The model under review builds one solid part; all positions refer to its coordinate system, in mm. Round coordinates to 2 decimals unless told otherwise and drop trailing zeros. Loops run counter-clockwise (first coordinate to the right, second up) from the corner with the lowest first, then second, coordinate; pieces in that order, holes last. Notation, with made-up numbers: (65.25, 47) -> (95.25, 47) arc R20 cw to (95.25, 51) -> close; hole circle Ø11 at (17.5, -1). An arc over 180 degrees is marked (long way). Write each question's results on one line, items separated by ' | '. Start each with the question number.
Item 1: Clearance check with flat-ended pins moving along their axes: pin 1 Ø0.5 at (x, z) = (0.5, 0.5) entering from +Y; pin 2 Ø0.9 at (x, z) = (15, 2) entering from -Y; pin 3 Ø0.9 at (x, z) = (-1, 2) entering from +Y. State where each tip first meets the part, or that it passes through.
Item 2: We need section D-D (y = -3.25). Give the boundary of the cut face in (x, z), and give its area (3 significant figures).
Item 3: We need section C-C (x = 11). Give the boundary of the cut face in (y, z).
Item 4: We need section A-A (y = 1). Give the boundary of the cut face in (x, z).
Item 5: For L1, parallel to Z at x = 20, y = 2; L2, parallel to X at y = 0.75, z = 1.15; L3, parallel to X at y = -0.25, z = 1.3, list the stretches that pass through material, from the lowest coordinate up. Write a range as from..to.
Item 6: We need section B-B (x = 15.25). Give the boundary of the cut face in (y, z).
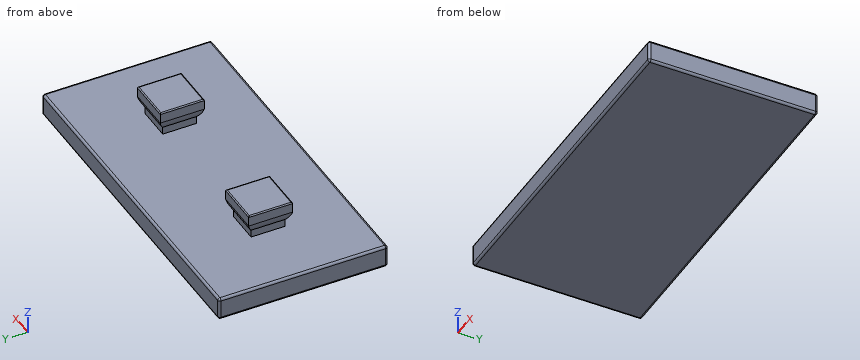
from build123d import *

# Parameters (mm, degrees)
SKETCH_1_W                      = 30
SKETCH_1_H                      = 15
EXTRUDE_1_DEPTH                 = 2
SKETCH_2_W                      = 3
SKETCH_2_H                      = 3
EXTRUDE_2_DEPTH                 = 1
EXTRUDE_3_DEPTH                 = 2
CUT_EXTRUDE_1_REACH             = 25.848
CUT_EXTRUDE_1_DIRECTION_2_REACH = 25.848
FILLET_1_R                      = 0.1
FILLET_1_OF_MIRROR_1_R          = 0.1
FILLET_3_R                      = 0.2


with BuildPart() as part:
    # Sketch 1 → Extrude 1 (new body)
    with BuildSketch(Plane.XY):
        with Locations((7.5, 0)):
            Rectangle(SKETCH_1_W, SKETCH_1_H)
    extrude(amount=-EXTRUDE_1_DEPTH)

    # Sketch 2 → Extrude 2 (add)
    with BuildSketch(Plane.XY):
        Rectangle(SKETCH_2_W, SKETCH_2_H)
    extrude_2 = extrude(amount=EXTRUDE_2_DEPTH)

    # Sketch 3 → Extrude 3 (add, symmetric)
    with BuildSketch(Plane(origin=(0, 0, 0), x_dir=(1, 0, 0), z_dir=(0, 1, 0))):
        with BuildLine():
            Line((-1.95, -2.5), (1.95, -2.5))
            Line((1.95, -2.5), (1.95, -1.555590279))
            ThreePointArc((1.95, -1.555590279), (1.780042303, -1.088161527), (1.5, -0.677124344))
            Line((1.5, -0.677124344), (-1.5, -0.677124344))
            ThreePointArc((-1.5, -0.677124344), (-1.780042303, -1.088161527), (-1.95, -1.555590279))
            Line((-1.95, -1.555590279), (-1.95, -2.5))
        make_face()
    extrude_3 = extrude(amount=EXTRUDE_3_DEPTH, both=True)

    # Sketch 4 → Cut-Extrude 1 (cut, up to next)
    with BuildSketch(Plane(origin=(0, 0, 0), x_dir=(0, 0, -1), z_dir=(1, 0, 0)), mode=Mode.PRIVATE) as cut_extrude_1_sk1:
        with BuildLine():
            Line((-2.5, 1.95), (-1.555590279, 1.95))
            ThreePointArc((-1.555590279, 1.95), (-1.088161527, 1.780042303), (-0.677124344, 1.5))
            Line((-0.677124344, 1.5), (-0.677124344, 2))
            Line((-0.677124344, 2), (-2.5, 2))
            Line((-2.5, 2), (-2.5, 1.95))
        make_face()
    cut_extrude_1_tool1 = extrude(cut_extrude_1_sk1.sketch, amount=-CUT_EXTRUDE_1_REACH, mode=Mode.PRIVATE) & part.part
    # Sketch 4 → Cut-Extrude 1 (cut, up to next)
    with BuildSketch(Plane(origin=(0, 0, 0), x_dir=(0, 0, -1), z_dir=(1, 0, 0)), mode=Mode.PRIVATE) as cut_extrude_1_sk2:
        with BuildLine():
            Line((-2.5, -2), (-0.677124344, -2))
            Line((-0.677124344, -2), (-0.677124344, -1.5))
            ThreePointArc((-0.677124344, -1.5), (-1.088161527, -1.780042303), (-1.555590279, -1.95))
            Line((-1.555590279, -1.95), (-2.5, -1.95))
            Line((-2.5, -1.95), (-2.5, -2))
        make_face()
    cut_extrude_1_tool2 = extrude(cut_extrude_1_sk2.sketch, amount=-CUT_EXTRUDE_1_REACH, mode=Mode.PRIVATE) & part.part
    cut_extrude_1_1 = cut_extrude_1_tool1.solids().sort_by_distance((0, 1.873038, 1.175075))[0]
    add(cut_extrude_1_1, mode=Mode.SUBTRACT)
    cut_extrude_1_2 = cut_extrude_1_tool2.solids().sort_by_distance((0, -1.873038, 1.175075))[0]
    add(cut_extrude_1_2, mode=Mode.SUBTRACT)
    cut_extrude_1 = cut_extrude_1_1 + cut_extrude_1_2  # Cut-Extrude 1 as one shape, for the pattern or mirror that repeats it

    # Sketch 4 → Cut-Extrude 1 direction 2 (cut, up to next)
    with BuildSketch(Plane(origin=(0, 0, 0), x_dir=(0, 0, -1), z_dir=(1, 0, 0)), mode=Mode.PRIVATE) as cut_extrude_1_direction_2_sk1:
        with BuildLine():
            Line((-2.5, 1.95), (-1.555590279, 1.95))
            ThreePointArc((-1.555590279, 1.95), (-1.088161527, 1.780042303), (-0.677124344, 1.5))
            Line((-0.677124344, 1.5), (-0.677124344, 2))
            Line((-0.677124344, 2), (-2.5, 2))
            Line((-2.5, 2), (-2.5, 1.95))
        make_face()
    cut_extrude_1_direction_2_tool1 = extrude(cut_extrude_1_direction_2_sk1.sketch, amount=CUT_EXTRUDE_1_DIRECTION_2_REACH, mode=Mode.PRIVATE) & part.part
    # Sketch 4 → Cut-Extrude 1 direction 2 (cut, up to next)
    with BuildSketch(Plane(origin=(0, 0, 0), x_dir=(0, 0, -1), z_dir=(1, 0, 0)), mode=Mode.PRIVATE) as cut_extrude_1_direction_2_sk2:
        with BuildLine():
            Line((-2.5, -2), (-0.677124344, -2))
            Line((-0.677124344, -2), (-0.677124344, -1.5))
            ThreePointArc((-0.677124344, -1.5), (-1.088161527, -1.780042303), (-1.555590279, -1.95))
            Line((-1.555590279, -1.95), (-2.5, -1.95))
            Line((-2.5, -1.95), (-2.5, -2))
        make_face()
    cut_extrude_1_direction_2_tool2 = extrude(cut_extrude_1_direction_2_sk2.sketch, amount=CUT_EXTRUDE_1_DIRECTION_2_REACH, mode=Mode.PRIVATE) & part.part
    cut_extrude_1_direction_2_1 = cut_extrude_1_direction_2_tool1.solids().sort_by_distance((0, 1.873038, 1.175075))[0]
    add(cut_extrude_1_direction_2_1, mode=Mode.SUBTRACT)
    cut_extrude_1_direction_2_2 = cut_extrude_1_direction_2_tool2.solids().sort_by_distance((0, -1.873038, 1.175075))[0]
    add(cut_extrude_1_direction_2_2, mode=Mode.SUBTRACT)
    cut_extrude_1_direction_2 = cut_extrude_1_direction_2_1 + cut_extrude_1_direction_2_2  # Cut-Extrude 1 direction 2 as one shape, for the pattern or mirror that repeats it

    # Fillet 1
    fillet_1_edges = [part.edges().sort_by_distance(p)[0] for p in [
        (-1.95, 0, 2.5),
        (1.95, 0, 2.5),
        (0, -1.95, 2.5),
        (0, 1.95, 2.5),
    ]]
    fillet(fillet_1_edges, radius=FILLET_1_R)

    # Mirror 1: Extrude 2, Extrude 3, Cut-Extrude 1, Cut-Extrude 1 direction 2 across plane
    add(extrude_2.mirror(Plane(origin=(7.5, 0, 0), x_dir=(0, 0, 1), z_dir=(1, 0, 0))))
    add(extrude_3.mirror(Plane(origin=(7.5, 0, 0), x_dir=(0, 0, 1), z_dir=(1, 0, 0))))
    add(cut_extrude_1.mirror(Plane(origin=(7.5, 0, 0), x_dir=(0, 0, 1), z_dir=(1, 0, 0))), mode=Mode.SUBTRACT)
    add(cut_extrude_1_direction_2.mirror(Plane(origin=(7.5, 0, 0), x_dir=(0, 0, 1), z_dir=(1, 0, 0))), mode=Mode.SUBTRACT)

    # Fillet 1 of Mirror 1
    fillet_1_of_mirror_1_edges = [part.edges().sort_by_distance(p)[0] for p in [
        (16.95, 0, 2.5),
        (13.05, 0, 2.5),
        (15, -1.95, 2.5),
        (15, 1.95, 2.5),
    ]]
    fillet(fillet_1_of_mirror_1_edges, radius=FILLET_1_OF_MIRROR_1_R)

    # Fillet 3
    fillet_3_edges = [part.edges().sort_by_distance(p)[0] for p in [
        (22.5, 0, -2),
        (7.5, 7.5, -2),
        (-7.5, 0, -2),
        (7.5, 7.5, 0),
        (22.5, 0, 0),
        (7.5, -7.5, 0),
        (-7.5, 0, 0),
        (7.5, -7.5, -2),
        (-7.5, 7.5, -1),
        (22.5, 7.5, -1),
        (22.5, -7.5, -1),
        (-7.5, -7.5, -1),
    ]]
    fillet(fillet_3_edges, radius=FILLET_3_R)


solid = part.part
Here are the results:
1) pin 1: stops at y = 1.56 | pin 2: stops at y = -1.95 | pin 3: stops at y = 1.95
2) outline: (-7.5, -1.8) arc R0.2 ccw to (-7.3, -2) -> (22.3, -2) arc R0.2 ccw to (22.5, -1.8) -> (22.5, -0.2) arc R0.2 ccw to (22.3, 0) -> (-7.3, 0) arc R0.2 ccw to (-7.5, -0.2) -> close | area: 60.0 mm2
3) outline: (-7.5, -1.8) arc R0.2 ccw to (-7.3, -2) -> (7.3, -2) arc R0.2 ccw to (7.5, -1.8) -> (7.5, -0.2) arc R0.2 ccw to (7.3, 0) -> (-7.3, 0) arc R0.2 ccw to (-7.5, -0.2) -> close
4) outline: (-7.5, -1.8) arc R0.2 ccw to (-7.3, -2) -> (22.3, -2) arc R0.2 ccw to (22.5, -1.8) -> (22.5, -0.2) arc R0.2 ccw to (22.3, 0) -> (16.5, 0) -> (16.5, 0.68) arc R2 ccw to (16.95, 1.56) -> (16.95, 2.4) arc R0.1 ccw to (16.85, 2.5) -> (13.15, 2.5) arc R0.1 ccw to (13.05, 2.4) -> (13.05, 1.56) arc R2 ccw to (13.5, 0.68) -> (13.5, 0) -> (1.5, 0) -> (1.5, 0.68) arc R2 ccw to (1.95, 1.56) -> (1.95, 2.4) arc R0.1 ccw to (1.85, 2.5) -> (-1.85, 2.5) arc R0.1 ccw to (-1.95, 2.4) -> (-1.95, 1.56) arc R2 ccw to (-1.5, 0.68) -> (-1.5, 0) -> (-7.3, 0) arc R0.2 ccw to (-7.5, -0.2) -> close
5) L1: z = -2..0 | L2: x = -1.81..1.81, 13.19..16.81 | L3: x = -1.87..1.87, 13.13..16.87
6) outline: (-7.5, -1.8) arc R0.2 ccw to (-7.3, -2) -> (7.3, -2) arc R0.2 ccw to (7.5, -1.8) -> (7.5, -0.2) arc R0.2 ccw to (7.3, 0) -> (1.5, 0) -> (1.5, 0.68) arc R2 ccw to (1.95, 1.56) -> (1.95, 2.4) arc R0.1 ccw to (1.85, 2.5) -> (-1.85, 2.5) arc R0.1 ccw to (-1.95, 2.4) -> (-1.95, 1.56) arc R2 ccw to (-1.5, 0.68) -> (-1.5, 0) -> (-7.3, 0) arc R0.2 ccw to (-7.5, -0.2) -> close
